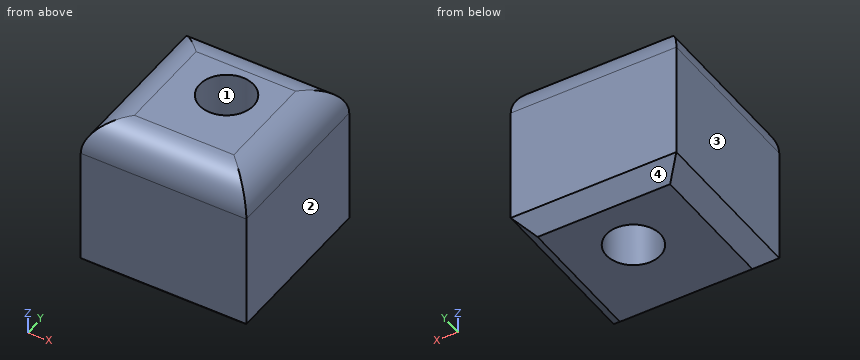
```python
from build123d import *

# Parameters (mm, degrees)
F0_W     = 100
F0_H     = 100
F1_DEPTH = 100
F2_R     = 20
F3_SIZE  = 10
F4_R     = 16.280572
F5_DEPTH = 173.821


with BuildPart() as f1:
    # F0 (on Top) → F1 (new body)
    with BuildSketch(Plane.XY):
        with Locations((3.83367, 5.873055)):
            Rectangle(F0_W, F0_H)
    extrude(amount=F1_DEPTH)

    # F2
    f2_edges = [f1.edges().sort_by_distance(p)[0] for p in [
        (-46.16633, 5.873055, 100),
        (3.83367, -44.126945, 100),
        (3.83367, 55.873055, 100),
        (53.83367, 5.873055, 100),
    ]]
    fillet(f2_edges, radius=F2_R)

    # F3
    f3_edges = [f1.edges().sort_by_distance(p)[0] for p in [
        (3.83367, -44.126945, 0),
        (53.83367, 5.873055, 0),
        (3.83367, 55.873055, 0),
        (-46.16633, 5.873055, 0),
    ]]
    chamfer(f3_edges, length=F3_SIZE)

    # F4 (on face) → F5 (cut)
    with BuildSketch(Plane.XY.offset(100)):
        with Locations((5.431035, 14.536005)):
            Circle(F4_R)
    extrude(amount=-F5_DEPTH, mode=Mode.SUBTRACT)


solid = f1.part
```
Source: CAD feature listing. Evaluate the final solid. Frame: model axes, mm. Face numbers are marked on the shaded views. Give positions to 0.01 mm unless a question says otherwise; leave off trailing zeros. Write each loop counter-clockwise with the first axis right and the second up, starting at its lowest first coordinate (ties: lowest second). Pieces come first, ordered by that corner, then holes. Notation, with made-up numbers: (23, -22.5) - (68, -22.5) arc R19 cw to (68, 0.5) - close; hole circle Ø5 at (30.5, 56). An arc over 180 degrees is marked (long way). One line per item, written item: value. Start each with the question number.
Q1. Section query B-B, the plane y = -10. Return the cut outline in (x, z).
Q2. Material intervals for probe 1 along X at (y, z) = (6.5, 43.5); probe 2 along X at (y, z) = (23.5, 9.5); probe 3 along Y at (x, z) = (-8.5, 82.5), sorted ascending. Write a range as from..to.
Q3. Draft query along X for the marked faces 1, 2, 3 and 4. Return one class per face: +X half, -X half, draft (parallel to the pull), parting line (faces both ways), or undercut.
Q4. Section query C-C, the plane z = 16. Return the cut outline in (x, y), then the cut area to 3 significant figures.
Q5. Section query A-A, the plane x = 6. Return the cut outline in (y, z), then the cut area to 3 significant figures.
Q6. Section query D-D, the plane y = 1. Return the cut outline in (x, z).
Answer:
1. outline: (-46.17, 10) - (-36.17, 0) - (43.83, 0) - (53.83, 10) - (53.83, 80) arc R20 ccw to (33.83, 100) - (-26.17, 100) arc R20 ccw to (-46.17, 80) - close
2. probe 1: x = -46.17..-8.73, 19.59..53.83
2. probe 2: x = -45.67..-8.16, 19.02..53.33
2. probe 3: y = -43.97..6.11, 22.96..55.72
3. face 1: undercut
3. face 2: +X half
3. face 3: -X half
3. face 4: draft
4. outline: (-46.17, -44.13) - (53.83, -44.13) - (53.83, 55.87) - (-46.17, 55.87) - close; hole circle Ø32.56 at (5.43, 14.54)
4. area: 9,170 mm2
5. outline: (-44.13, 10) - (-34.13, 0) - (-1.73, 0) - (-1.73, 100) - (-24.13, 100) arc R20 ccw to (-44.13, 80) - close; (30.81, 0) - (45.87, 0) - (55.87, 10) - (55.87, 80) arc R20 ccw to (35.87, 100) - (30.81, 100) - close
5. area: 6,470 mm2
6. outline: (-46.17, 10) - (-36.17, 0) - (-3.62, 0) - (-3.62, 100) - (-26.17, 100) arc R20 ccw to (-46.17, 80) - close; (14.48, 0) - (43.83, 0) - (53.83, 10) - (53.83, 80) arc R20 ccw to (33.83, 100) - (14.48, 100) - close
